from build123d import *

# Parameters (mm, degrees)
SKETCH1_R           = 4
SKETCH1_R_2         = 2
SKETCH1_R_3         = 3.17
BOSS_EXTRUDE1_DEPTH = 2


with BuildPart() as part:
    # Sketch1 → Boss-Extrude1 (new body)
    with BuildSketch(Plane(origin=(0, 0, 0), x_dir=(0, 0, -1), z_dir=(1, 0, 0))):
        with BuildLine():
            Line((54.519367594, -39.969907591), (54.519367594, 2.030092409))
            Line((54.519367594, 2.030092409), (44.519367594, 2.030092409))
            Line((44.519367594, 2.030092409), (44.519367594, 3.030092409))
            ThreePointArc((44.519367594, 3.030092409), (44.226474376, 3.73719919), (43.519367594, 4.030092409))
            Line((43.519367594, 4.030092409), (30.519367594, 4.030092409))
            ThreePointArc((30.519367594, 4.030092409), (29.812260813, 3.73719919), (29.519367594, 3.030092409))
            Line((29.519367594, 3.030092409), (29.519367594, 2.030092409))
            Line((29.519367594, 2.030092409), (24.519367594, 2.030092409))
            Line((24.519367594, 2.030092409), (24.519367594, 47.030092409))
            Line((24.519367594, 47.030092409), (16.268858723, 47.030092409))
            Line((16.268858723, 47.030092409), (16.268858723, 48.030092409))
            ThreePointArc((16.268858723, 48.030092409), (15.975965504, 48.73719919), (15.268858723, 49.030092409))
            Line((15.268858723, 49.030092409), (-23.230123534, 49.030092409))
            ThreePointArc((-23.230123534, 49.030092409), (-23.937230315, 48.73719919), (-24.230123534, 48.030092409))
            Line((-24.230123534, 48.030092409), (-24.230123534, 47.030092409))
            Line((-24.230123534, 47.030092409), (-27.680632406, 47.030092409))
            Line((-27.680632406, 47.030092409), (-27.680632406, 39.030092409))
            Line((-27.680632406, 39.030092409), (-29.680632406, 39.030092409))
            Line((-29.680632406, 39.030092409), (-29.680632406, 47.030092409))
            Line((-29.680632406, 47.030092409), (-35.480632406, 47.030092409))
            Line((-35.480632406, 47.030092409), (-35.480632406, -39.969907591))
            Line((-35.480632406, -39.969907591), (-24.230123534, -39.969907591))
            Line((-24.230123534, -39.969907591), (-24.230123534, -40.969907591))
            ThreePointArc((-24.230123534, -40.969907591), (-23.937230315, -41.677014372), (-23.230123534, -41.969907591))
            Line((-23.230123534, -41.969907591), (34.268858723, -41.969907591))
            ThreePointArc((34.268858723, -41.969907591), (34.975965504, -41.677014372), (35.268858723, -40.969907591))
            Line((35.268858723, -40.969907591), (35.268858723, -39.969907591))
            Line((35.268858723, -39.969907591), (54.519367594, -39.969907591))
        make_face()
        with Locations((36.233846968, -22.469907591)):
            Circle(SKETCH1_R, mode=Mode.SUBTRACT)
        with Locations((49.233846968, -9.469907591)):
            Circle(SKETCH1_R_2, mode=Mode.SUBTRACT)
        with Locations((23.233846968, -35.469907591)):
            Circle(SKETCH1_R_2, mode=Mode.SUBTRACT)
        with Locations((-19.680632406, 3.530092409)):
            Circle(SKETCH1_R_3, mode=Mode.SUBTRACT)
        with Locations((8.276607281, -9.469907591)):
            Circle(SKETCH1_R_3, mode=Mode.SUBTRACT)
    extrude(amount=BOSS_EXTRUDE1_DEPTH)


solid = part.part
Build history of the part. All positions in model axes, mm. A direction names the side the tool comes from. Round coordinates to 2 decimals unless told otherwise and drop trailing zeros. Order: outer loops, then holes, each group sorted by start corner. A loop starts at its lowest first (then second) coordinate and runs counter-clockwise, first axis right, second up. Notation, with made-up numbers: M 15.25,24.5 L 68.25,24.5 A15 ccw 68.25,30.5 Z; hole C 16.5,88.5 d8. An arc over 180 degrees is marked long. Use CSV: the item, a comma, the result in double quotes. Start each with the question number.
(1) Cut at B-B on y = 41. List the corners of the cut face in (x, z).
(2) Mould opens along Z. For faces 1 (the face through (1, 49.03, 4)), 2 (the face through (0.986, -9.382, -47.236)), 3 (the face through (1, 43, 27.681)), 4 (the face through (1, 4, 35.481)) say: +Z half, -Z half, draft (parallel to the pull), parting line (faces both ways), or undercut.
(3) Cut at A-A on z = -23. List the corners of the cut face in (x, y), then the cut area to 3 significant figures.
(4) Drill centre lines: probe 1 along Y at (x, z) = (1.15, -42); probe 2 along Y at (x, z) = (0.1, -38); probe 3 along Z at (x, y) = (1.4, -24.5). Where is each one in solid material? Low to high.
(5) Cut at D-D on y = 19.5. List the corners of the cut face in (x, z), then the cut area to 3 significant figures.
(6) Tool access for faces 5 (the face through (1, 43, 29.681)), 6 (the face through (1, 4.03, -37)), 7 (the face through (1, 47.03, 33)), 8 (the face through (1, -39.97, 30)): list every direction of +Z, -Z, +X, -X, +Y, -Y with a clear straight run to the whole face (end or side of a thin tool).
(7) Cut at C-C on x = 0.75. State how many separate pieces and enclosed holes the cut face has, then the cut area to 3 significant figures.
(8) Flat gauge pins, fed straight in: P1, Ø0.6, axis at x = 0.5, z = -39, coming from the +Y side; P2, Ø4, axis at y = 27, z = -27, coming from the +X side; P3, Ø0.6, axis at x = 1, z = -40.5, coming from the -Y side; P4, Ø0.5, axis at x = 0.5, y = -40.5, coming from the -Z side. Where does each tip first touch, or does it go through?
Findings:
1,outline,"M 0,-24.52 L 2,-24.52 L 2,27.68 L 0,27.68 Z; M 0,29.68 L 2,29.68 L 2,35.48 L 0,35.48 Z"
2,face 1,"draft"
2,face 2,"undercut"
2,face 3,"undercut"
2,face 4,"+Z half"
3,outline,"M 0,-41.97 L 2,-41.97 L 2,-37.46 L 0,-37.46 Z; M 0,-33.48 L 2,-33.48 L 2,47.03 L 0,47.03 Z"
3,area,"170 mm^2"
4,probe 1,"y = -39.97 to 4.03"
4,probe 2,"y = -39.97 to -26.06, -18.88 to 4.03"
4,probe 3,"z = -54.52 to -39.68, -32.79 to 35.48"
5,outline,"M 0,-24.52 L 2,-24.52 L 2,35.48 L 0,35.48 Z"
5,area,"120 mm^2"
6,face 5,"+X, -X, +Y"
6,face 6,"-Z, +X, -X, +Y"
6,face 7,"+Z, +X, -X, +Y"
6,face 8,"+Z, +X, -X, -Y"
7,separate pieces,"1"
7,enclosed holes,"5"
7,area,"6,550 mm^2"
8,P1,"stops at y = 4.03"
8,P2,"passes through"
8,P3,"stops at y = -39.97"
8,P4,"stops at z = -35.27"
